The model under review builds one solid part; all positions refer to its coordinate system, in mm. A direction names the side the tool comes from. Coordinates: 2 decimals unless noted, no trailing zeros. Loops run counter-clockwise (first coordinate to the right, second up) from the corner with the lowest first, then second, coordinate; pieces in that order, holes last. Notation, with made-up numbers: (84, -21) - (135, -21) arc R24 ccw to (135, -3) - close; hole circle Ø5 at (14, 54.5). An arc over 180 degrees is marked (long way). Use a Markdown table: item, result. Add a question column.
1) Add section C-C, the plane z = 6.25. Give the boundary of the cut face in (x, y), and give its area (3 significant figures).
2) Add section A-A, the plane y = 30.5. Give the boundary of the cut face in (x, z), and give its area (3 significant figures).
3) For faces 4 (the flat face through (35, 3, 7)), 5 (the cylindrical face through (63.39, 6.42, 6.53)), 6 (the flat face through (35, 58, 1.6)), 7 (the flat face through (67, 63, 7)), list the 3-axis set-ups (+Z, -Z, +X, -X, +Y, -Y) from which the entire face can be reached by the end or side of a thin tool; tool diameter is ignored.
4) To check wall thickness, follow L1, parallel to Y at x = 46.5, z = 0.5; L2, parallel to X at y = 80, z = 7.75; L3, parallel to Y at x = 34, z = 5. State the ranges of each line that lie inside material, in increasing order. Write a range as [from, to].
5) Add section B-B, the plane x = 20. Give the boundary of the cut face in (y, z).
6) The part is to be moulded in two halves that separate along Y. For faces 1 (the cylindrical face through (5.9, 56.93, 2.46)), 2 (the cylindrical face through (6.61, 108.58, 6.53)), 3 (the cylindrical face through (6.42, 6.61, 6.53)), say which applies: pulls with the +Y half, pulls with the -Y half, needs draft (parallel to the pull), parting line crosses it, or undercut.
7) Clearance check with flat-ended pins moving along their axes: pin 1 (1.5 mm diameter, centred on x = 8.5, z = 1.5, fed in from +Y); pin 2 (10 mm diameter, centred on x = 52, y = 37.5, fed in from +Z); pin 3 (1.5 mm diameter, centred on x = 41.5, z = 4, fed in from +Y). State where each tip first meets the part, or that it passes through.
```python
from build123d import *

# Parameters (mm, degrees)
PAD_DEPTH       = 1.6
PAD001_DEPTH    = 10
SKETCH004_R     = 1
POCKET_DEPTH    = 67.001
POCKET001_DEPTH = 5
CHAMFER_SIZE    = 1
FILLET_R        = 3
POCKET002_DEPTH = 5


with BuildPart() as part:
    # Sketch → Pad (new body)
    with BuildSketch(Plane.XY):
        with BuildLine():
            Line((12, 0), (58, 0))
            ThreePointArc((58, 0), (66.485281, 3.514719), (70, 12))
            Line((70, 12), (70, 115))
            Line((70, 115), (12, 115))
            ThreePointArc((12, 115), (3.514719, 111.485281), (0, 103))
            Line((0, 103), (0, 12))
            ThreePointArc((0, 12), (3.514719, 3.514719), (12, 0))
        make_face()
    extrude(amount=PAD_DEPTH)

    # Sketch001 → Pad001 (new body)
    with BuildSketch(Plane.XY.offset(1.6)):
        with BuildLine():
            Line((15, 3), (55, 3))
            ThreePointArc((55, 3), (63.485281, 6.514719), (67, 15))
            Line((67, 15), (67, 112))
            Line((67, 112), (15, 112))
            ThreePointArc((15, 112), (6.514719, 108.485281), (3, 100))
            Line((3, 100), (3, 15))
            ThreePointArc((3, 15), (6.514719, 6.514719), (15, 3))
        make_face()
        with BuildLine():
            Line((17, 5), (53, 5))
            ThreePointArc((53, 5), (61.485281, 8.514719), (65, 17))
            Line((65, 17), (65, 110))
            Line((65, 110), (17, 110))
            ThreePointArc((17, 110), (8.514719, 106.485281), (5, 98))
            Line((5, 98), (5, 17))
            ThreePointArc((5, 17), (8.514719, 8.514719), (17, 5))
        make_face(mode=Mode.SUBTRACT)
    extrude(amount=PAD001_DEPTH)

    # Sketch004 → Pocket (cut, through all)
    with BuildSketch(Plane.YZ.offset(67)):
        with Locations((-62, 7.1)):
            Circle(SKETCH004_R)
    extrude(amount=-POCKET_DEPTH, mode=Mode.SUBTRACT)

    # Sketch005 → Pocket001 (cut)
    with BuildSketch(Plane.XY.offset(1.6)):
        with BuildLine():
            Line((25, 96), (47, 96))
            ThreePointArc((48.5, 94.5), (48.06066, 95.56066), (47, 96))
            Line((48.5, 94.5), (48.5, 82.5))
            ThreePointArc((47, 81), (48.06066, 81.43934), (48.5, 82.5))
            Line((47, 81), (25, 81))
            ThreePointArc((23.5, 82.5), (23.93934, 81.43934), (25, 81))
            Line((23.5, 82.5), (23.5, 94.5))
            ThreePointArc((25, 96), (23.93934, 95.56066), (23.5, 94.5))
        make_face()
    extrude(amount=-POCKET001_DEPTH, mode=Mode.SUBTRACT)

    # Chamfer
    chamfer_edges = [part.edges().sort_by_distance(p)[0] for p in [
        (48.5, 88.5, 1.6),
        (48.06066, 95.56066, 1.6),
        (36, 96, 1.6),
        (23.93934, 95.56066, 1.6),
        (23.5, 88.5, 1.6),
        (23.93934, 81.43934, 1.6),
        (36, 81, 1.6),
        (48.06066, 81.43934, 1.6),
    ]]
    chamfer(chamfer_edges, length=CHAMFER_SIZE)

    # Fillet
    fillet_edges = [part.edges().sort_by_distance(p)[0] for p in [
        (41, 110, 1.6),
        (8.514719, 106.485281, 1.6),
        (65, 63.5, 1.6),
        (5, 57.5, 1.6),
        (8.514719, 8.514719, 1.6),
        (35, 5, 1.6),
    ]]
    fillet(fillet_edges, radius=FILLET_R)

    # Sketch006 → Pocket002 (cut)
    with BuildSketch(Plane(origin=(0, 112, 0), x_dir=(-1, 0, 0), z_dir=(0, 1, 0))):
        with BuildLine():
            ThreePointArc((-55, 18), (-59, 22), (-63, 18))
            Line((-63, 18), (-63, 8))
            ThreePointArc((-63, 8), (-59, 4), (-55, 8))
            Line((-55, 18), (-55, 8))
        make_face()
    extrude(amount=-POCKET002_DEPTH, mode=Mode.SUBTRACT)


solid = part.part
```
From the geometry:
| question | item | result |
|---|---|---|
| 1 | outline | (3, 15) arc R12 ccw to (15, 3) - (55, 3) arc R12 ccw to (67, 15) - (67, 112) - (62.6, 112) - (62.6, 110) - (65, 110) - (65, 17) arc R12 cw to (53, 5) - (17, 5) arc R12 cw to (5, 17) - (5, 98) arc R12 cw to (17, 110) - (55.4, 110) - (55.4, 112) - (15, 112) arc R12 ccw to (3, 100) - close |
| 1 | area | 662 mm^2 |
| 2 | outline | (0, 0) - (70, 0) - (70, 1.6) - (67, 1.6) - (67, 11.6) - (65, 11.6) - (65, 4.6) arc R3 cw to (62, 1.6) - (8, 1.6) arc R3 cw to (5, 4.6) - (5, 11.6) - (3, 11.6) - (3, 1.6) - (0, 1.6) - close |
| 2 | area | 156 mm^2 |
| 3 | face 4 | +Z, +X, -X, -Y |
| 3 | face 5 | +Z, +X, -Y |
| 3 | face 6 | +Z |
| 3 | face 7 | +Z, +X, +Y, -Y |
| 4 | L1 | y = [0, 81], [96, 115] |
| 4 | L2 | x = [3, 5], [65, 67] |
| 4 | L3 | y = [3, 5], [110, 112] |
| 5 | outline | (0, 0) - (115, 0) - (115, 1.6) - (112, 1.6) - (112, 11.6) - (110, 11.6) - (110, 4.6) arc R3 cw to (107, 1.6) - (8, 1.6) arc R3 cw to (5, 4.6) - (5, 11.6) - (3, 11.6) - (3, 1.6) - (0, 1.6) - close |
| 6 | face 1 | undercut |
| 6 | face 2 | pulls with the +Y half |
| 6 | face 3 | pulls with the -Y half |
| 7 | pin 1 | stops at y = 114.68 |
| 7 | pin 2 | stops at z = 1.6 |
| 7 | pin 3 | stops at y = 112 |
